Read the model definition and answer for the solid it produces. Units are mm, in the model's axes. A direction names the side the tool comes from. Round coordinates to 2 decimals unless told otherwise and drop trailing zeros. Order: outer loops, then holes, each group sorted by start corner. A loop starts at its lowest first (then second) coordinate and runs counter-clockwise, first axis right, second up. Notation, with made-up numbers: (-18.75, 36.25) -> (38.25, 36.25) arc R28 ccw to (38.25, 71.25) -> close; hole circle Ø2 at (45, -25). An arc over 180 degrees is marked (long way). Use a Markdown table: item, result. Add a question column.
1. The mould has two halves that part along Y. Classify faces 1 (the face through (19, 78, 25)), 2 (the face through (42.049, 56.214, 6.409)), 3 (the face through (55.482, 82.871, 6.591)), 4 (the face through (-45.951, 56.214, 6.409)): +Y half, -Y half, draft (parallel to the pull), parting line (faces both ways), or undercut.
2. For faces 5 (the face through (-7.5, 19, 38)), 6 (the face through (41, 52, 13)), 7 (the face through (-1, 0, 38)), determine the directions among +Z, -Z, +X, -X, +Y, -Y from which every point of the face is accessible in a straight line to the end or side of a thin tool.
3. Section A-A, the plane z = 49 is taken. Give the vertices of the cut face in (x, y).
4. Section B-B, the plane y = 38.5 is taken. Give the vertices of the cut face in (x, z), then the cut area to 3 significant figures.
5. Given pin 1 (7 mm diameter, centred on y = 18.5, z = 34.5, fed in from -X); pin 2 (11.5 mm diameter, centred on x = 5.5, y = 83.5, fed in from +Z); pin 3 (14.5 mm diameter, centred on x = 44, z = 53, fed in from +Y); pin 4 (6 mm diameter, centred on x = -50.5, y = 77.5, fed in from +Z), each flat-ended and moving along its own axis, determine where each tip first touches the part or whether it passes through.
6. Consider L1, parallel to X at y = 5.25, z = 53; L2, parallel to Z at x = 44, y = 9; L3, parallel to X at y = 65, z = 9. Determine where each line is inside the solid, lowest interval first. Write a range as [from, to].
7. Section D-D, the plane z = 18.5 is taken. Give the vertices of the cut face in (x, y), then the cut area to 3 significant figures.
8. Section C-C, the plane x = 44 is taken. Give the vertices of the cut face in (y, z), then the cut area to 3 significant figures.
```python
from build123d import *

# Parameters (mm, degrees)
SKETCH1_W               = 63
SKETCH1_H               = 13
BOSS_EXTRUDE1_DEPTH     = 78
BOSS_EXTRUDE2_DEPTH     = 51
BOSS_EXTRUDE3_DEPTH     = 13
BOSS_EXTRUDE5_DEPTH     = 38
FILLET1_R               = 25
CUT_EXTRUDE1_DEPTH      = 135.733069437
CUT_EXTRUDE1_DEPTH_BACK = 135.733069437
SKETCH3_R               = 9
CUT_EXTRUDE2_DEPTH      = 135.733069437
CUT_EXTRUDE2_DEPTH_BACK = 135.733069437
SKETCH2_R               = 9


with BuildPart() as part:
    # Sketch1 → Boss-Extrude1 (new body)
    with BuildSketch(Plane.XY):
        with Locations((-31.5, 6.5)):
            Rectangle(SKETCH1_W, SKETCH1_H)
        with Locations((31.5, 6.5)):
            Rectangle(SKETCH1_W, SKETCH1_H)
    extrude(amount=BOSS_EXTRUDE1_DEPTH)



with BuildPart() as body_2:
    # Sketch1<3> → Boss-Extrude2 (new body)
    with BuildSketch(Plane.XY):
        with BuildLine():
            ThreePointArc((-19, 67.248076809), (-22.706848309, 40.540600405), (0, 26))
            Line((0, 26), (0, 35))
            ThreePointArc((0, 35), (-16, 51), (0, 67))
            Line((0, 67), (0, 76))
            ThreePointArc((0, 76), (-10.459399595, 73.706848309), (-19, 67.248076809))
        make_face()
        with BuildLine():
            Line((0, 35), (0, 26))
            ThreePointArc((0, 26), (17.67766953, 33.32233047), (25, 51))
            ThreePointArc((25, 51), (23.452078799, 59.660254038), (19, 67.248076809))
            ThreePointArc((19, 67.248076809), (10.459399595, 73.706848309), (0, 76))
            Line((0, 76), (0, 67))
            ThreePointArc((0, 67), (11.313708499, 62.313708499), (16, 51))
            ThreePointArc((16, 51), (11.313708499, 39.686291501), (0, 35))
        make_face()
    extrude(amount=BOSS_EXTRUDE2_DEPTH)


with BuildPart() as part_1:
    add(part.part)

    add(body_2.part)  # Boss-Extrude3 merges body 2
    # Sketch1<5> → Boss-Extrude3 (add)
    with BuildSketch(Plane.XY):
        with BuildLine():
            Line((0, 13), (63, 13))
            Line((63, 13), (63, 90))
            Line((63, 90), (19, 90))
            Line((19, 90), (19, 67.248076809))
            ThreePointArc((19, 67.248076809), (23.452078799, 59.660254038), (25, 51))
            ThreePointArc((25, 51), (17.67766953, 33.32233047), (0, 26))
            Line((0, 26), (0, 13))
        make_face()
        with BuildLine():
            Line((-63, 13), (0, 13))
            Line((0, 13), (0, 26))
            ThreePointArc((0, 26), (-22.706848309, 40.540600405), (-19, 67.248076809))
            Line((-19, 67.248076809), (-19, 90))
            Line((-19, 90), (-63, 90))
            Line((-63, 90), (-63, 13))
        make_face()
    extrude(amount=BOSS_EXTRUDE3_DEPTH)

    # Sketch1<7> → Boss-Extrude5 (add)
    with BuildSketch(Plane.XY):
        with BuildLine():
            Line((-19, 90), (-19, 67.248076809))
            ThreePointArc((-19, 67.248076809), (-10.459399595, 73.706848309), (0, 76))
            Line((0, 76), (0, 81))
            ThreePointArc((0, 81), (-6.363961031, 83.636038969), (-9, 90))
            Line((-9, 90), (-19, 90))
        make_face()
        with BuildLine():
            Line((19, 67.248076809), (19, 90))
            Line((19, 90), (9, 90))
            ThreePointArc((9, 90), (6.363961031, 83.636038969), (0, 81))
            Line((0, 81), (0, 76))
            ThreePointArc((0, 76), (10.459399595, 73.706848309), (19, 67.248076809))
        make_face()
    extrude(amount=BOSS_EXTRUDE5_DEPTH)

    # Fillet1
    fillet1_edges = [part_1.edges().sort_by_distance(p)[0] for p in [
        (-63, 90, 6.5),
        (63, 90, 6.5),
    ]]
    fillet(fillet1_edges, radius=FILLET1_R)

    # Sketch3 → Cut-Extrude1 (cut, two sides: drawn at the far end of the back side and taken through both)
    with BuildSketch(Plane(origin=(0, 0, 0), x_dir=(1, 0, 0), z_dir=(0, 1, 0)).offset(-CUT_EXTRUDE1_DEPTH_BACK)):
        with Locations(Location((-44, -53, 0), (0, 0, 270))):
            Circle(SKETCH3_R)
        with Locations(Location((44, -53, 0), (0, 0, 270))):
            Circle(SKETCH3_R)
    extrude(amount=CUT_EXTRUDE1_DEPTH + CUT_EXTRUDE1_DEPTH_BACK, mode=Mode.SUBTRACT)

    # Sketch2 → Cut-Extrude2 (cut, two sides: drawn at the far end of the back side and taken through both)
    with BuildSketch(Plane.XY.offset(-CUT_EXTRUDE2_DEPTH_BACK)):
        with Locations((-44, 65)):
            Circle(SKETCH2_R)
        with Locations((44, 65)):
            Circle(SKETCH2_R)
    extrude(amount=CUT_EXTRUDE2_DEPTH + CUT_EXTRUDE2_DEPTH_BACK, mode=Mode.SUBTRACT)

    # Sketch13 → Loft1 section 0
    with BuildSketch(Plane(origin=(-7.5, 0, 0), x_dir=(0, 0, -1), z_dir=(1, 0, 0))):
        with BuildLine():
            Line((-78, 13), (-13, 13))
            Line((-13, 13), (-13, 27.151519965))
            Line((-13, 27.151519965), (-51, 27.151519965))
            Line((-51, 27.151519965), (-78, 13))
        make_face()
    # Sketch5 → Loft1 section 1
    with BuildSketch(Plane(origin=(0, 0, 0), x_dir=(0, 0, -1), z_dir=(1, 0, 0))):
        with BuildLine():
            Line((-78, 13), (-51, 26.066063348))
            Line((-51, 26.066063348), (-13, 26))
            Line((-13, 26), (-13, 13))
            Line((-13, 13), (-78, 13))
        make_face()
    # Sketch12 → Loft1 section 2
    with BuildSketch(Plane(origin=(7.5, 0, 0), x_dir=(0, 0, -1), z_dir=(1, 0, 0))):
        with BuildLine():
            Line((-51, 27.151519965), (-78, 13))
            Line((-78, 13), (-13, 13))
            Line((-13, 13), (-13, 27.151519965))
            Line((-13, 27.151519965), (-51, 27.151519965))
        make_face()
    loft()


solid = part_1.part
```
Verdict:
| question | item | result |
|---|---|---|
| 1 | face 1 | draft |
| 1 | face 2 | undercut |
| 1 | face 3 | +Y half |
| 1 | face 4 | undercut |
| 2 | face 5 | +Z, -X |
| 2 | face 6 | +Z, +X |
| 2 | face 7 | +Z, -Z, +X, -X, -Y |
| 3 | outline | (-63, 0) -> (-52.06, 0) -> (-52.06, 13) -> (-63, 13) -> close; (-35.94, 0) -> (35.94, 0) -> (35.94, 13) -> (7.5, 13) -> (7.5, 27.15) arc R25 ccw (long way) to (-7.5, 27.15) -> (-7.5, 13) -> (-35.94, 13) -> close; (52.06, 0) -> (63, 0) -> (63, 13) -> (52.06, 13) -> close; hole circle Ø32 at (0, 51) |
| 4 | outline | (-63, 0) -> (-9.99, 0) -> (-9.99, 51) -> (-21.65, 51) -> (-21.65, 13) -> (-63, 13) -> close; (9.99, 0) -> (63, 0) -> (63, 13) -> (21.65, 13) -> (21.65, 51) -> (9.99, 51) -> close |
| 4 | area | 2,260 mm2 |
| 5 | pin 1 | stops at x = -7.5 |
| 5 | pin 2 | stops at z = 38 |
| 5 | pin 3 | passes through |
| 5 | pin 4 | stops at z = 13 |
| 6 | L1 | x = [-63, -53], [-35, 35], [53, 63] |
| 6 | L2 | z = [0, 44], [62, 78] |
| 6 | L3 | x = [-63, -53], [-35, -7.75], [7.75, 35], [53, 63] |
| 7 | outline | (-63, 0) -> (63, 0) -> (63, 13) -> (7.5, 13) -> (7.5, 27.15) arc R25 ccw to (19, 67.25) -> (19, 90) -> (9, 90) arc R9 cw to (-9, 90) -> (-19, 90) -> (-19, 67.25) arc R25 ccw to (-7.5, 27.15) -> (-7.5, 13) -> (-63, 13) -> close; hole circle Ø32 at (0, 51) |
| 7 | area | 3,500 mm2 |
| 8 | outline | (0, 0) -> (56, 0) -> (56, 13) -> (13, 13) -> (13, 44) -> (0, 44) -> close; (0, 62) -> (13, 62) -> (13, 78) -> (0, 78) -> close; (74, 0) -> (89.27, 0) -> (89.27, 13) -> (74, 13) -> close |
| 8 | area | 1,540 mm2 |
